```python
from build123d import *

# Parameters (mm, degrees)
SKETCH1_W           = 30.2
SKETCH1_H           = 51.3
BOSS_EXTRUDE1_DEPTH = 5
BOSS_EXTRUDE2_DEPTH = 27.5
SKETCH3_W           = 30.2
SKETCH3_H           = 5
BOSS_EXTRUDE3_DEPTH = 7
SKETCH4_W           = 30.2
SKETCH4_H           = 5
BOSS_EXTRUDE4_DEPTH = 7
SKETCH5_W           = 30.2
SKETCH5_H           = 65.3
SKETCH5_W_2         = 20.2
SKETCH5_H_2         = 55.3
BOSS_EXTRUDE5_DEPTH = 8.7
FILLET1_R           = 5
FILLET2_R           = 2.5
FILLET3_R           = 2.5


with BuildPart() as part:
    # Sketch1 → Boss-Extrude1 (new body)
    with BuildSketch(Plane(origin=(0, 0, 0), x_dir=(1, 0, 0), z_dir=(0, 1, 0))):
        Rectangle(SKETCH1_W, SKETCH1_H)
    extrude(amount=BOSS_EXTRUDE1_DEPTH)

    # Sketch2 → Boss-Extrude2 (add)
    with BuildSketch(Plane(origin=(0, 5, 0), x_dir=(1, 0, 0), z_dir=(0, 1, 0))):
        Polygon((10.1, -20.65), (5.1, -20.65), (5.1, -25.65), (15.1, -25.65), (15.1, 25.65), (-15.1, 25.65), (-15.1, -25.65), (-5.1, -25.65), (-5.1, -20.65), (-10.1, -20.65), (-10.1, 20.65), (10.1, 20.65), align=None)
    extrude(amount=BOSS_EXTRUDE2_DEPTH)

    # Sketch3 → Boss-Extrude3 (add)
    with BuildSketch(Plane.XY.offset(25.65)):
        with Locations((0, 30)):
            Rectangle(SKETCH3_W, SKETCH3_H)
    extrude(amount=BOSS_EXTRUDE3_DEPTH)

    # Sketch4 → Boss-Extrude4 (add)
    with BuildSketch(Plane(origin=(0, 0, -25.65), x_dir=(-1, 0, 0), z_dir=(0, 0, -1))):
        with Locations((0, 30)):
            Rectangle(SKETCH4_W, SKETCH4_H)
    extrude(amount=BOSS_EXTRUDE4_DEPTH)

    # Sketch5 → Boss-Extrude5 (add)
    with BuildSketch(Plane(origin=(0, 32.5, 0), x_dir=(1, 0, 0), z_dir=(0, 1, 0))):
        Rectangle(SKETCH5_W, SKETCH5_H)
        Rectangle(SKETCH5_W_2, SKETCH5_H_2, mode=Mode.SUBTRACT)
    extrude(amount=BOSS_EXTRUDE5_DEPTH)

    # Fillet1
    fillet1_edges = [part.edges().sort_by_distance(p)[0] for p in [
        (15.1, 13.75, 25.65),
        (-15.1, 13.75, 25.65),
        (-15.1, 34.35, 32.65),
        (15.1, 34.35, 32.65),
        (-15.1, 13.75, -25.65),
        (15.1, 13.75, -25.65),
        (15.1, 34.35, -32.65),
        (-15.1, 34.35, -32.65),
    ]]
    fillet(fillet1_edges, radius=FILLET1_R)

    # Fillet2
    fillet2_edges = [part.edges().sort_by_distance(p)[0] for p in [
        (-5.1, 16.25, 25.65),
        (5.1, 16.25, 25.65),
        (-5.1, 18.75, 20.65),
        (5.1, 18.75, 20.65),
    ]]
    fillet(fillet2_edges, radius=FILLET2_R - 0.0001)  # a hair under: the kernel refuses the full size

    # Fillet3
    fillet3_edges = [part.edges().sort_by_distance(p)[0] for p in [
        (-5.1, 30, 25.65),
        (5.1, 30, 25.65),
    ]]
    fillet(fillet3_edges, radius=FILLET3_R - 0.0001)  # a hair under: the kernel refuses the full size


solid = part.part
```
Work out the finished part from the listing and answer in its coordinate system (mm). A direction names the side the tool comes from. Round coordinates to 2 decimals unless told otherwise and drop trailing zeros. Loops run counter-clockwise (first coordinate to the right, second up) from the corner with the lowest first, then second, coordinate; pieces in that order, holes last. Notation, with made-up numbers: (32, 84) -> (87, 84) arc R4 cw to (87, 90) -> close; hole circle Ø2 at (19, 46.5). An arc over 180 degrees is marked (long way). Write each question's results on one line, items separated by ' | '. Start each with the question number.
1. For a pull along Z with two mould halves and no side action, classify faces 5 (the face through (0, 19, -20.65)), 6 (the face through (0, 34, -32.65)), 7 (the face through (0, 5, 2)), 8 (the face through (0, 0, 0)) as +Z half, -Z half, draft (parallel to the pull), parting line (faces both ways), or undercut.
2. Find the intervals of material crossed by probe 1 along X at (y, z) = (5.5, 10.5); probe 2 along Z at (x, y) = (-3, 35); probe 3 along Z at (x, y) = (10, 17), in increasing order. Write a range as from..to.
3. Section C-C (x = 9) is taken. Determine the outline of the cut face in (y, z), plus the area to 4 significant figures.
4. Section B-B (z = -0.5) is taken. Determine the outline of the cut face in (x, y).
5. Given pin 1 Ø2 at (x, y) = (10.5, 13) entering from +Z; pin 2 Ø1 at (y, z) = (14.5, -23.5) entering from -X; pin 3 Ø5.5 at (x, z) = (-2, -24) entering from +Y, each flat-ended and moving along its own axis, determine where each tip first touches the part or whether it passes through.
6. A tool of negligible diameter and unlimited length cuts with its end or side. For faces 1 (the face through (-5.852, 16.408, 24.937)), 2 (the face through (-13.67, 13.56, 24.15)), 3 (the face through (13.67, 13.94, 24.15)), 4 (the face through (0, 32.5, 26)), from which of +Z, -Z, +X, -X, +Y, -Y can it reach the whole face along a straight path? Write none if from no direction.
Evaluation:
1) face 5: undercut | face 6: -Z half | face 7: undercut | face 8: draft
2) probe 1: x = -15.1..-10.1, 10.1..15.1 | probe 2: z = -32.65..-27.65, 27.65..32.65 | probe 3: z = -25.65..-20.65, 20.65..25.65
3) outline: (0, -25.65) -> (27.5, -25.65) -> (27.5, -32.65) -> (41.2, -32.65) -> (41.2, -27.65) -> (32.5, -27.65) -> (32.5, -20.65) -> (5, -20.65) -> (5, 20.65) -> (32.5, 20.65) -> (32.5, 27.65) -> (41.2, 27.65) -> (41.2, 32.65) -> (27.5, 32.65) -> (27.5, 25.65) -> (0, 25.65) -> close | area: 688.5 mm2
4) outline: (-15.1, 0) -> (15.1, 0) -> (15.1, 41.2) -> (10.1, 41.2) -> (10.1, 5) -> (-10.1, 5) -> (-10.1, 41.2) -> (-15.1, 41.2) -> close
5) pin 1: stops at z = 25.65 | pin 2: stops at x = -14.51 | pin 3: stops at y = 32.5
6) face 1: +Z | face 2: +Z, -X, -Y | face 3: +Z, +X, -Y | face 4: +Y
